```python
from build123d import *

# Parameters (mm, degrees)
F1_DEPTH = 190.5
F2_R     = 25.4
F3_R     = 5.08
F5_DEPTH = 177.8


with BuildPart() as f1:
    # F0 (on Top) → F1 (new body)
    with BuildSketch(Plane.XY):
        Polygon((0, 0), (0, 127), (-381, 63.5), (-381, 0), align=None)
        Polygon((0, -127), (0, 0), (-381, 0), (-381, -63.5), align=None)
    extrude(amount=F1_DEPTH)

    # F2
    f2_edges = [f1.edges().sort_by_distance(p)[0] for p in [
        (-190.5, -95.25, 190.5),
        (-190.5, 95.25, 190.5),
    ]]
    fillet(f2_edges, radius=F2_R)

    # F3
    f3_edges = [f1.edges().sort_by_distance(p)[0] for p in [
        (-381, 0, 190.5),
    ]]
    fillet(f3_edges, radius=F3_R)

    # F4 (on Top) → F5 (cut)
    with BuildSketch(Plane.XY):
        Polygon((-374.832104, -57.15), (0, -120.65), (0, 120.65), (-374.832104, 57.15), (-374.832104, 0), align=None)
    extrude(amount=F5_DEPTH, mode=Mode.SUBTRACT)


solid = f1.part
```
For this review, take the finished solid that the model builds, in its own axes (mm). A direction names the side the tool comes from. Give positions to 0.01 mm unless a question says otherwise; leave off trailing zeros. Write each loop counter-clockwise with the first axis right and the second up, starting at its lowest first coordinate (ties: lowest second). Pieces come first, ordered by that corner, then holes.
Item 1: The part is to be moulded in two halves that separate along Y. For faces 1 (the face through (-234, -84, 0)), 2 (the face through (-191.5, 87.7, 182.9)), 3 (the face through (-190.04, -88.456, 87.655)), 4 (the face through (-374.832, 1, 88)), say which applies: +Y half, -Y half, draft (parallel to the pull), parting line (faces both ways), or undercut.
Item 2: Wall thickness on probe 1 along Z at (x, y) = (-82, 12); probe 2 along Y at (x, z) = (-33.5, 27); probe 3 along Y at (x, z) = (-204, 168): over which ranges is each line inside the solid? List them lowest first.
Item 3: Machinability: for faces 5 (the face through (-148, 2, 177.8)), 6 (the face through (-381, 1, 91)), which of the approach directions +Z, -Z, +X, -X, +Y, -Y give a long, thin tool a straight path to every point of the face, cutting with its end or side? Answer none if there is none.
Item 4: Take a section at A-A (y = -1). Give the boundary of the cut face in (x, z).
Item 5: Take a section at B-B (z = 73). Give the boundary of the cut face in (x, y), and give its area (3 significant figures).
Item 6: Insertion check: P1, Ø3, axis at y = 2.5, z = 114.5, coming from the +X side; P2, Ø1, axis at x = -170, z = 51, coming from the -Y side; P3, Ø12, axis at x = -281.5, y = 86.5, coming from the +Z side; P4, Ø1, axis at x = -295, y = 13.5, coming from the -Z side. Each pin has a flat end and moves straight along its axis. Give the tip position at first contact, or say it passes through.
Established:
1. face 1: draft
1. face 2: +Y half
1. face 3: undercut
1. face 4: undercut
2. probe 1: z = 177.8 to 190.5
2. probe 2: y = -121.42 to -114.97, 114.97 to 121.42
2. probe 3: y = -92.83 to -86.09, 86.09 to 92.83
3. face 5: -Z, +X
3. face 6: +Z, -Z, -X, +Y, -Y
4. outline: (-381, 0) - (-374.83, 0) - (-374.83, 177.8) - (0, 177.8) - (0, 190.5) - (-375.92, 190.5) arc R5.08 ccw to (-381, 185.42) - close
5. outline: (-381, -59.2) arc R5.08 ccw to (-376.76, -64.21) - (0, -127) - (0, -120.65) - (-374.83, -57.15) - (-374.83, 57.15) - (0, 120.65) - (0, 127) - (-376.76, 64.21) arc R5.08 ccw to (-381, 59.2) - close
5. area: 5,930 mm2
6. P1: stops at x = -374.83
6. P2: stops at y = -98.75
6. P3: passes through
6. P4: stops at z = 177.8
